Part model, mm, in its own coordinate system. Face numbers are marked on the shaded views. A direction names the side the tool comes from. Coordinates: 2 decimals unless noted, no trailing zeros. Order: outer loops, then holes, each group sorted by start corner. A loop starts at its lowest first (then second) coordinate and runs counter-clockwise, first axis right, second up.
1) Tool access for the marked faces 1, 2, 3, 4 and 5: list every direction of +Z, -Z, +X, -X, +Y, -Y with a clear straight run to the whole face (end or side of a thin tool).
2) Pin check, flat tips, straight feed: pin 1 Ø3.5 at (y, z) = (25.5, 1) entering from -X; pin 2 Ø0.5 at (x, z) = (1.5, 1) entering from -Y; pin 3 Ø1.9 at (y, z) = (15.5, 5) entering from +X. Stop position of each tip, or through.
3) Cut at A-A (y = 9.5). List the corners of the cut face in (x, z).
4) Wall check: L1, parallel to X at y = 15.5, z = 2.5; L2, parallel to Y at x = 11, z = 3.5 (3 decimals); L3, parallel to Y at x = 22, z = 7 (3 decimals). Give the ranges that are in metal, low to high.
5) Cut at C-C (x = 9.5). List the corners of the cut face in (y, z) (3 decimals).
6) Cut at D-D (z = 2.5). List the corners of the cut face in (x, y), and give its area (3 significant figures).
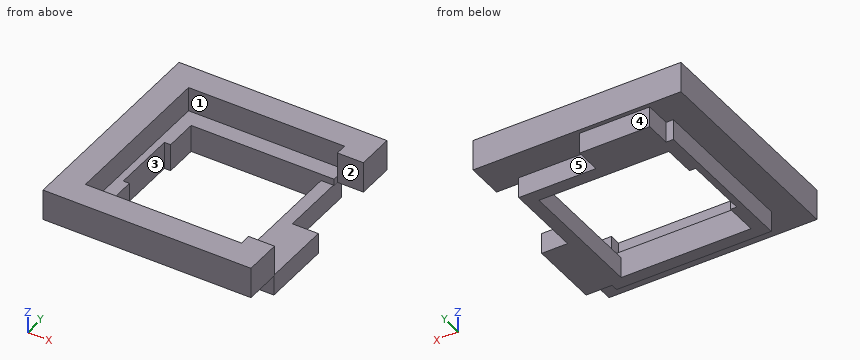
Autodesk Inventor part; units mm, degrees
ref_plane "YZ Plane" through (0, 0, 0) normal (1, 0, 0) x (0, 1, 0)
ref_plane "XZ Plane" through (0, 0, 0) normal (0, 1, 0) x (-1, 0, 0)
ref_plane "XY Plane" through (0, 0, 0) normal (0, 0, 1) x (1, 0, 0)
sketch "Sketch1" plane through (0, 0, 0) normal (0, 0, 1) x (1, 0, 0)
  line L0 (0, 0) -> (0, 24) construction
  line L1 (0, 24) -> (1.113, 24) construction
  line L2 (1.113, 24) -> (1.113, 28) construction
  line L3 (1.113, 28) -> (12.113, 28) construction
  line L4 (12.113, 28) -> (12.113, 24) construction
  line L5 (12.113, 24) -> (24, 24) construction
  line L6 (24, 24) -> (24, 12.1) construction
  line L7 (24, 12.1) -> (28, 12.1) construction
  line L8 (28, 12.1) -> (28, 1.1) construction
  line L9 (28, 1.1) -> (24, 1.1) construction
  line L10 (24, 1.1) -> (24, 0) construction
  line L11 (24, 0) -> (0, 0) construction
  line L12 (12.013, 27.9) -> (1.213, 27.9)
  line L13 (1.213, 27.9) -> (1.213, 23.9)
  line L14 (1.213, 23.9) -> (0.1, 23.9)
  line L15 (0.1, 23.9) -> (0.1, 0.1)
  line L16 (0.1, 0.1) -> (23.9, 0.1)
  line L17 (23.9, 0.1) -> (23.9, 1.2)
  line L18 (23.9, 1.2) -> (27.9, 1.2)
  line L19 (27.9, 1.2) -> (27.9, 12)
  line L20 (27.9, 12) -> (23.9, 12)
  line L21 (23.9, 12) -> (23.9, 23.9)
  line L22 (23.9, 23.9) -> (12.013, 23.9)
  line L23 (12.013, 23.9) -> (12.013, 27.9)
  circle A0 centre (-1.945, 26.005) radius 1.548
  circle A1 centre (26.025, 26.005) radius 1.548
  circle A2 centre (-2.025, -2.005) radius 1.548
  circle A3 centre (26.025, -2.005) radius 1.548
  line L24 (0.1, 23.9) -> (23.9, 0.1) construction
  line L25 (23.9, 23.9) -> (0.1, 0.1) construction
  line L26 (-1.945, 26.005) -> (26.025, -2.005) construction
  line L27 (-2.025, -2.005) -> (26.025, 26.005) construction
  line L28 (2, 22) -> (22, 22)
  line L29 (22, 22) -> (22, 2)
  line L30 (22, 2) -> (2, 2)
  line L31 (2, 2) -> (2, 22) construction
  line L32 (2, 17) -> (1.05, 17)
  line L33 (1.05, 17) -> (1.05, 7)
  line L34 (1.05, 7) -> (2, 7)
  line L35 (2, 17) -> (2, 22)
  line L36 (2, 7) -> (2, 2)
  point P0 (12, 12)
  point P1 (1.05, 12)
  point P2 (12, 12)
  dimension "d0" = 24
  dimension "d1" = 1.113
  dimension "d2" = 4
  dimension "d3" = 11
  dimension "d4" = 11.887
  dimension "d5" = 11.9
  dimension "d6" = 4
  dimension "d7" = 11
  dimension "d8" = 1.1
  dimension "d9" = 0.1
  dimension "d10" = 3.096
  dimension "d11" = 27.97
  dimension "d12" = 28.01
  dimension "d15" = 20
  dimension "d16" = 0.95
  dimension "d17" = 10
extrude "Extrusion1" add sketch "Sketch1" along normal blind 3.2 contours L23 L22 L21 L20 L19 L18 L17 L16 L15 L14 L13 L12
sketch "Sketch2" plane through (0, 0, 3.2) normal (0, 0, 1) x (1, 0, 0)
  line L0 (0, 24.535) -> (24, 24.535)
  line L1 (24, 24.535) -> (24, -0.535) construction
  line L2 (24, -0.535) -> (0, -0.535)
  line L3 (0, -0.535) -> (0, 24.535)
  line L4 (22, 22) -> (22, 2)
  line L5 (1.3564, 23.1456) -> (22, 2) construction
  line L6 (22, 22) -> (2.0347, 2) construction
  line L7 (2, 22) -> (22, 22)
  line L8 (28, 28.535) -> (-4, 28.535)
  line L9 (-4, 28.535) -> (-4, -4.535)
  line L10 (-4, -4.535) -> (28, -4.535)
  line L11 (28, -4.535) -> (28, 28.535)
  line L12 (24, 1.2) -> (28, 1.2)
  line L13 (24, 22.8) -> (28, 22.8)
  line L14 (24, 24.535) -> (24, 22.8)
  line L15 (24, -0.535) -> (24, 1.2)
  line L16 (23.9, 0.1) -> (23.9, 1.2)
  point P0 (0, 0)
  point P1 (12, 24.535)
  point P2 (12, 22)
  point P3 (24, 12)
  point P4 (22, 12)
  dimension "d18" = 25.07
  dimension "d19" = 24
  dimension "d20" = 4
  dimension "d21" = 1.735
  dimension "d22" = 1.735
extrude "Extrusion2" add sketch "Sketch2" along normal blind 4.75 contours L3 L2 L15 L12 L11 L10 L9 L8 L13 L14 L0
sketch "Sketch3" plane through (0, 0, 3.2) normal (0, 0, 1) x (1, 0, 0)
  line L0 (28, 1.2) -> (24, 1.2)
  line L1 (24, 1.2) -> (24, -0.535)
  line L2 (24, -0.535) -> (0, -0.535)
  line L3 (0, -0.535) -> (0, 24.535)
  line L4 (0, 24.535) -> (24, 24.535)
  line L5 (24, 24.535) -> (24, 22.8)
  line L6 (24, 22.8) -> (28, 22.8)
  line L7 (28, 22.8) -> (28, 28.535)
  line L8 (28, 28.535) -> (-4, 28.535)
  line L9 (-4, 28.535) -> (-4, -4.535)
  line L10 (-4, -4.535) -> (28, -4.535)
  line L11 (28, -4.535) -> (28, 1.2)
  line L12 (12.013, 24.535) -> (1.213, 24.535)
  line L13 (1.213, 24.535) -> (1.213, 23.9)
  line L14 (1.213, 23.9) -> (0.1, 23.9)
  line L15 (0.1, 23.9) -> (0.1, 0.1)
  line L16 (0.1, 0.1) -> (23.9, 0.1)
  line L17 (23.9, 0.1) -> (23.9, 1.2)
  line L18 (23.9, 1.2) -> (24, 1.2)
  line L19 (24, 1.2) -> (27.9, 1.2)
  line L20 (27.9, 1.2) -> (27.9, 12)
  line L21 (27.9, 12) -> (23.9, 12)
  line L22 (23.9, 12) -> (23.9, 23.9)
  line L23 (23.9, 23.9) -> (12.013, 23.9)
  line L24 (12.013, 23.9) -> (12.013, 24.535)
  line L25 (22, 22) -> (22, 2)
  line L26 (22, 2) -> (2, 2)
  line L27 (2, 2) -> (2, 7)
  line L28 (2, 7) -> (1.05, 7)
  line L29 (1.05, 7) -> (1.05, 17)
  line L30 (1.05, 17) -> (2, 17)
  line L31 (2, 17) -> (2, 22)
  line L32 (2, 22) -> (22, 22)
  line L33 (0, 24.535) -> (1.213, 24.535)
  line L34 (0, 24.535) -> (24, 24.535)
  line L35 (24, 24.535) -> (24, 22.8)
  line L36 (2, 22) -> (22, 22)
  line L37 (12.013, 24.535) -> (24, 24.535)
  line L38 (24, 24.535) -> (24, 22)
  line L39 (2, 17) -> (2, 22)
  line L40 (24, 22) -> (2, 22)
  line L41 (2, 22) -> (2, 17)
  line L42 (1.05, 7) -> (1.05, 17)
  line L43 (2, 17) -> (1.05, 17)
  line L44 (1.05, 17) -> (1.05, 7)
  line L45 (2, 2) -> (2, 7)
  line L46 (1.05, 7) -> (2, 7)
  line L47 (2, 7) -> (2, 2)
  line L48 (2, 2) -> (24, 2)
  line L49 (24, 2) -> (24, 1.2)
  line L50 (24, 1.2) -> (24, -0.535)
  line L51 (24, 1.2) -> (24, -0.535)
  line L52 (24, -0.535) -> (0, -0.535)
  line L53 (0, -0.535) -> (0, 24.535)
  line L54 (0, 24.535) -> (0, -0.535)
  line L55 (24, -0.535) -> (0, -0.535)
  line L56 (0, -0.535) -> (24, -0.535)
  line L57 (24, -0.535) -> (24, 2)
  point P0 (0, 0)
  point P1 (23.9, 22)
extrude "Extrusion3" add sketch "Sketch3" along normal blind 1 contours L1 L2 L3 L4 L13 L14 L15 L16 L17 L18 | L18 L17 L16 L15 L14 L13 L4 L24 L23 L22 L40 L32 L31 L30 L29 L28 L27 L26 L48 L49 | L22 L23 L24 L4 L5 L38 L40
properties part number "Camera Mod"
Geometry check:
1. face 1: +Z
1. face 2: +Z, -Z, +X
1. face 3: +Z, -Z
1. face 4: -Z, +X, -X, +Y
1. face 5: -Z, +X, +Y
2. pin 1: stops at x = 0.1
2. pin 2: stops at y = 0.1
2. pin 3: stops at x = 1.05
3. outline: (-4, 3.2) - (0.1, 3.2) - (0.1, 0) - (1.05, 0) - (1.05, 4.2) - (0, 4.2) - (0, 7.95) - (-4, 7.95) - close; (22, 0) - (27.9, 0) - (27.9, 3.2) - (22, 3.2) - close
4. L1: x = 0.1 to 1.05, 22 to 23.9
4. L2: y = -4.535 to 2, 22 to 28.535
4. L3: y = -4.535 to -0.535, 24.535 to 28.535
5. outline: (-4.535, 3.2) - (0.1, 3.2) - (0.1, 0) - (2, 0) - (2, 4.2) - (-0.535, 4.2) - (-0.535, 7.95) - (-4.535, 7.95) - close; (22, 0) - (27.9, 0) - (27.9, 3.2) - (28.535, 3.2) - (28.535, 7.95) - (24.535, 7.95) - (24.535, 4.2) - (22, 4.2) - close
6. outline: (0.1, 0.1) - (23.9, 0.1) - (23.9, 1.2) - (27.9, 1.2) - (27.9, 12) - (23.9, 12) - (23.9, 23.9) - (12.01, 23.9) - (12.01, 27.9) - (1.21, 27.9) - (1.21, 23.9) - (0.1, 23.9) - close; hole (1.05, 7) - (2, 7) - (2, 2) - (22, 2) - (22, 22) - (2, 22) - (2, 17) - (1.05, 17) - close
6. area: 243 mm2
